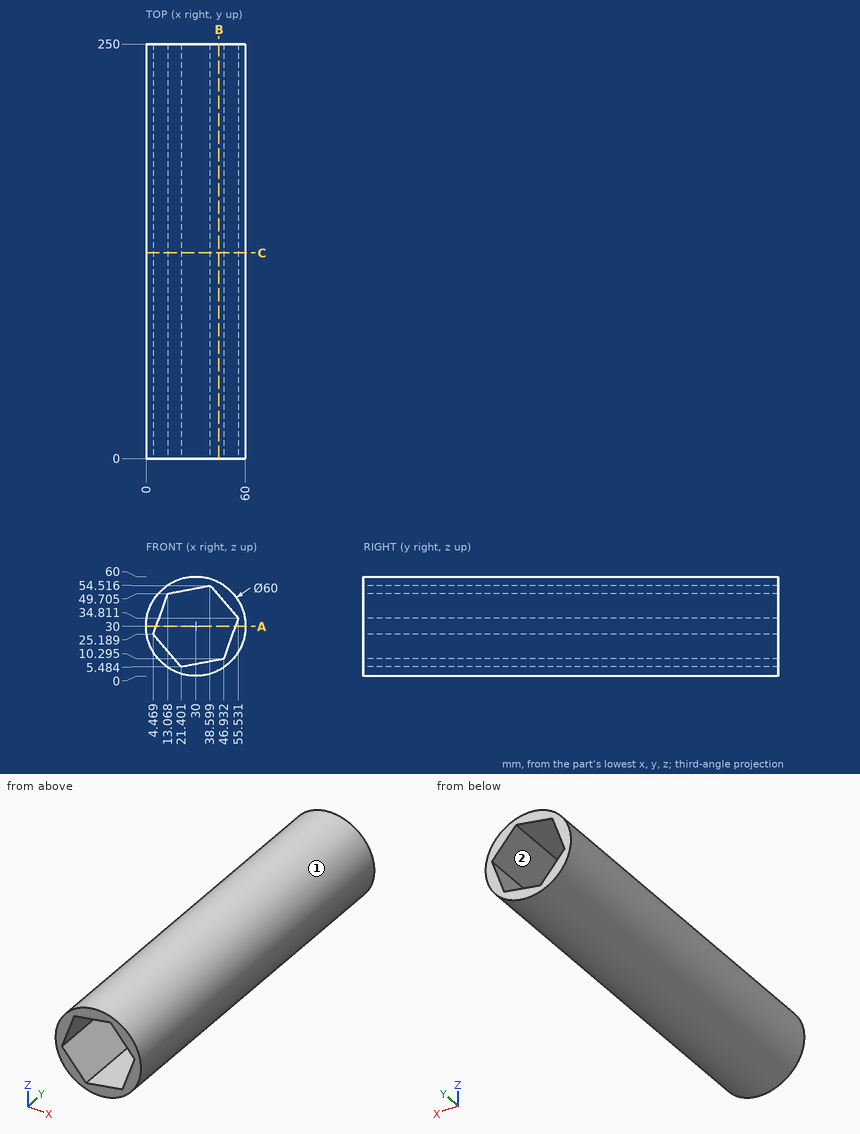
Input: dimensioned drawing with shaded views. Units: mm. Origin: part minimum x, y, z. Coordinates: 2 decimals unless noted, no trailing zeros. Order: outer loops, then holes, each group sorted by start corner. A loop starts at its lowest first (then second) coordinate and runs counter-clockwise, first axis right, second up.
(1) Section query A-A (z = 30). Return the cut outline in (x, y), plus the area to 3 significant figures.
(2) Draft query along X for the marked faces 1 and 2. Return one class per face: pulls with the +X half, pulls with the -X half, needs draft (parallel to the pull), parting line crosses it, or undercut.
(3) First-contact query: pin 1 (1.5 mm diameter, centred on x = 42.5, y = 151.5, fed in from +Z); pin 2 (6 mm diameter, centred on x = 13.5, y = 93.5, fed in from -Z); pin 3 (5 mm diameter, centred on x = 17.5, y = 71.5, fed in from +Z) (1 decimal). Flat tips, straight axial feed; report the tip coordinate or a pass-through.
(4) Material intervals for probe 1 along X at (y, z) = (160.5, 18) (1 decimal); probe 2 along Z at (x, y) = (37, 189) (1 decimal); probe 3 along Z at (x, y) = (37.5, 212), sorted ascending.
(5) Section query C-C (y = 124). Return the cut outline in (x, z) (1 decimal).
(6) Section query B-B (x = 44). Return the cut outline in (y, z).
Solution:
1. outline: (0, 0) - (6.16, 0) - (6.16, 250) - (0, 250) - close; (53.84, 0) - (60, 0) - (60, 250) - (53.84, 250) - close
1. area: 3,080 mm2
2. face 1: parting line crosses it
2. face 2: undercut
3. pin 1: stops at z = 57.6
3. pin 2: stops at z = 3.21
3. pin 3: stops at z = 58.3
4. probe 1: x = 2.5 to 10.6, 49.6 to 57.5
4. probe 2: z = 0.8 to 8.4, 54.2 to 59.2
4. probe 3: z = 0.95 to 8.52, 54.31 to 59.05
5. outline: circle Ø60 at (30, 30); hole (4.5, 25.2) - (21.4, 5.5) - (46.9, 10.3) - (55.5, 34.8) - (38.6, 54.5) - (13.1, 49.7) - close
6. outline: (0, 3.47) - (250, 3.47) - (250, 9.74) - (0, 9.74) - close; (0, 48.23) - (250, 48.23) - (250, 56.53) - (0, 56.53) - close
